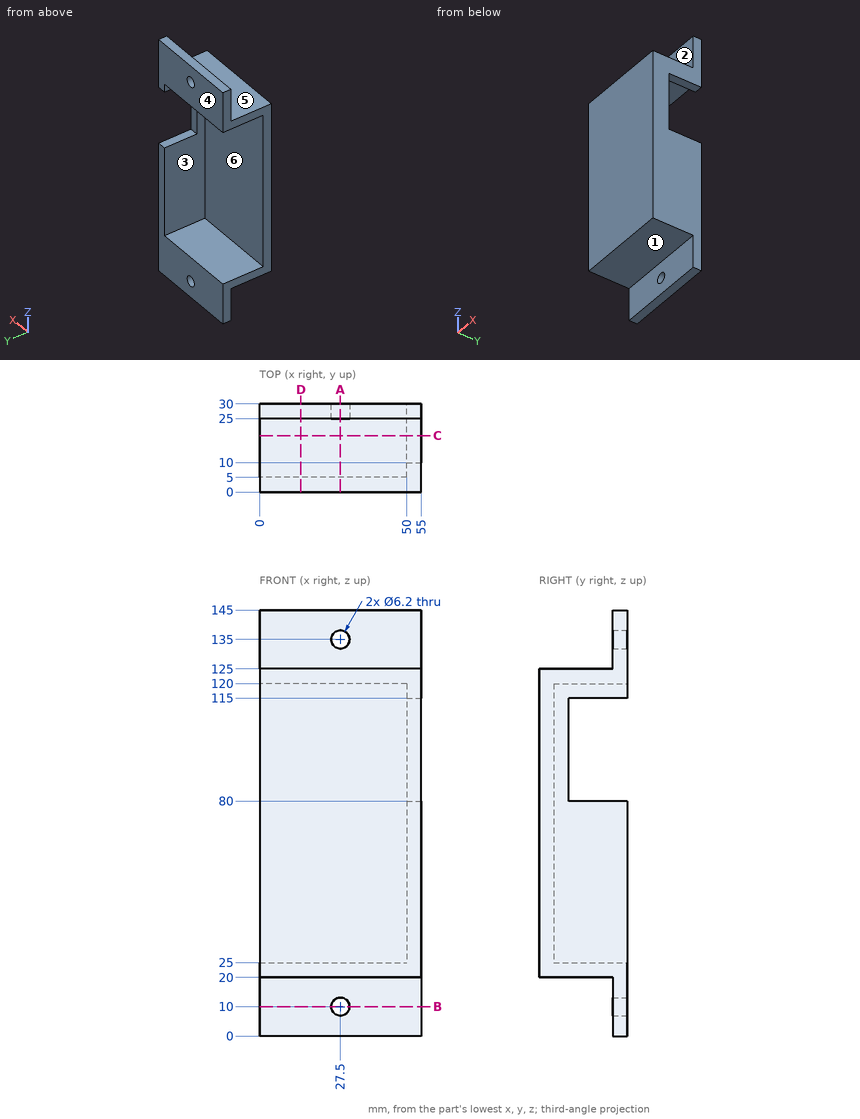
Answer from the drawing. Dimensions are ordinates in mm from the lowest x, y and z of the part. A direction names the side the tool comes from. Coordinates: 2 decimals unless noted, no trailing zeros. Order: outer loops, then holes, each group sorted by start corner. A loop starts at its lowest first (then second) coordinate and runs counter-clockwise, first axis right, second up. Notation, with made-up numbers: (56, 34) - (82, 34) arc R23 cw to (82, 62) - close; hole circle Ø9 at (-8, -16). An arc over 180 degrees is marked (long way). Answer as a JSON object with one key per item and string values. Group by question number.
Item 1: Section C-C (y = 19.25) is taken. Give the vertices of the cut face in (x, z).
Item 2: The mould has two halves that part along Z. Classify the marked faces 4, 5 and 6: +Z half, -Z half, draft (parallel to the pull), parting line (faces both ways), or undercut.
Item 3: Section A-A (x = 27.5) is taken. Give the vertices of the cut face in (y, z).
Item 4: Section D-D (x = 14) is taken. Give the vertices of the cut face in (y, z).
Item 5: A tool of negligible diameter and unlimited length cuts with its end or side. For the marked faces 1, 2 and 3, from which of +Z, -Z, +X, -X, +Y, -Y can it reach the whole face along a straight path? Write none if from no direction.
Item 6: Flat-ended cylindrical pins translate along their axes: P1, Ø2.5, axis at x = 52.5, y = 19.5, coming from the +Z side; P2, Ø5.5, axis at x = 53.5, z = 103, coming from the +Y side; P3, Ø6, axis at x = 19.5, z = 12.5, coming from the -Y side; P4, Ø1.5, axis at x = 44.5, z = 120.5, coming from the -Y side. Find the tip coordinate at first contact, or state that the pin passes through.
Item 7: Consider probe 1 along Z at (x, y) = (27.5, 27.6); probe 2 along Z at (x, y) = (30, 15); probe 3 along X at (y, z) = (26.5, 10). Determine where each line is inside the solid, lowest interval first. Write a range as from..to.
Item 8: Section B-B (z = 10) is taken. Give the vertices of the cut face in (x, y).
Results are:
{
 "1": {"outline": "(0, 20) - (55, 20) - (55, 80) - (50, 80) - (50, 25) - (0, 25) - close; (0, 120) - (50, 120) - (50, 115) - (55, 115) - (55, 125) - (0, 125) - close"},
 "2": {"face 4": "draft", "face 5": "+Z half", "face 6": "undercut"},
 "3": {"outline": "(0, 20) - (25, 20) - (25, 13.1) - (30, 13.1) - (30, 25) - (5, 25) - (5, 120) - (30, 120) - (30, 131.9) - (25, 131.9) - (25, 125) - (0, 125) - close; (25, 0) - (30, 0) - (30, 6.9) - (25, 6.9) - close; (25, 138.1) - (30, 138.1) - (30, 145) - (25, 145) - close"},
 "4": {"outline": "(0, 20) - (25, 20) - (25, 0) - (30, 0) - (30, 25) - (5, 25) - (5, 120) - (30, 120) - (30, 145) - (25, 145) - (25, 125) - (0, 125) - close"},
 "5": {"face 1": "-Z, +X, -X, -Y", "face 2": "+Z, +X, -X, -Y", "face 3": "-X, +Y"},
 "6": {"P1": "stops at z = 125", "P2": "stops at y = 10", "P3": "stops at y = 25", "P4": "stops at y = 0"},
 "7": {"probe 1": "z = 0..6.9, 13.1..25, 120..131.9, 138.1..145", "probe 2": "z = 20..25, 120..125", "probe 3": "x = 0..24.4, 30.6..55"},
 "8": {"outline": "(0, 25) - (24.4, 25) - (24.4, 30) - (0, 30) - close; (30.6, 25) - (55, 25) - (55, 30) - (30.6, 30) - close"}
}
